Build history of the part. All positions in model axes, mm. A direction names the side the tool comes from. Round coordinates to 2 decimals unless told otherwise and drop trailing zeros. Order: outer loops, then holes, each group sorted by start corner. A loop starts at its lowest first (then second) coordinate and runs counter-clockwise, first axis right, second up. Notation, with made-up numbers: (71.25, -30.75) - (93.25, -30.75) arc R25 cw to (93.25, 7.25) - close; hole circle Ø1 at (41.25, 63). An arc over 180 degrees is marked (long way). One line per question, with ' | ' between items. Start each with the question number.
from build123d import *

# Parameters (mm, degrees)
SKETCH_1_R          = 11
SKETCH_1_R_2        = 5
EXTRUDE_1_DEPTH     = 6
SKETCH_2_R          = 9.499624375
SKETCH_2_R_2        = 7
CUT_EXTRUDE_1_DEPTH = 0.6
SKETCH_3_R          = 9.950876812
SKETCH_3_R_2        = 7
CUT_EXTRUDE_2_DEPTH = 0.6
CHAMFER_1_SIZE      = 0.2


with BuildPart() as part:
    # 草图1 → 凸台-拉伸1 (new body)
    with BuildSketch(Plane(origin=(0, 0, 0), x_dir=(0, 0, -1), z_dir=(1, 0, 0))):
        Circle(SKETCH_1_R)
        Circle(SKETCH_1_R_2, mode=Mode.SUBTRACT)
    extrude(amount=EXTRUDE_1_DEPTH)

    # 草图2 → 切除-拉伸1 (cut)
    with BuildSketch(Plane(origin=(6, 0, 0), x_dir=(0, 0, -1), z_dir=(1, 0, 0))):
        with Locations((-0.000375625, 0)):
            Circle(SKETCH_2_R)
        with Locations((-0.000375625, 0)):
            Circle(SKETCH_2_R_2, mode=Mode.SUBTRACT)
    extrude(amount=-CUT_EXTRUDE_1_DEPTH, mode=Mode.SUBTRACT)

    # 草图3 → 切除-拉伸2 (cut)
    with BuildSketch(Plane.ZY):
        with Locations((0.450876812, 0)):
            Circle(SKETCH_3_R)
        with Locations((0.450876812, 0)):
            Circle(SKETCH_3_R_2, mode=Mode.SUBTRACT)
    extrude(amount=-CUT_EXTRUDE_2_DEPTH, mode=Mode.SUBTRACT)

    # 倒角1
    chamfer_1_edges = [part.edges().sort_by_distance(p)[0] for p in [
        (0, 0, 11),
        (6, 0, 11),
        (0, 0, 5),
        (6, 0, 5),
    ]]
    chamfer(chamfer_1_edges, length=CHAMFER_1_SIZE)


solid = part.part
Item 1: Pull direction Z, two halves, no side cores. Call faces 1 (the face through (2.96, -10.74, 2.38)), 2 (the face through (6, -10, 0)), 3 (the face through (0.296, 9.866, -0.845)): released by +Z, released by -Z, zero draft, split by the parting line, or undercut.
Item 2: Wall check: line 1 along X through (y, z) = (-9, 2.5); line 2 along X through (y, z) = (4.25, -5.5); line 3 along Y through (x, z) = (0.5, -1). Give the ranges that are in metal, low to high. Write a range as [from, to].
Item 3: Slice it at C-C (x = 4.5). Write the cut outline in (y, z).
Item 4: 3-axis set-ups, long thin cutter, end or side, ignore diameter. For faces 4 (the face through (0, -1.5, 5.2)), 5 (the face through (0.3, 4.73, -4.71)), 6 (the face through (5.704, -3.638, -8.775)): which of +Z, -Z, +X, -X, +Y, -Y reach the whole face in a straight line?
Item 5: Pin check, flat tip, straight feed: pin 1 (8 mm diameter, centred on y = 0, z = 0, fed in from +X). Stop position of the tip, or through.
A:
1) face 1: split by the parting line | face 2: zero draft | face 3: undercut
2) line 1: [0.6, 5.4] | line 2: [0.6, 6] | line 3: [-10.95, -9.84], [-6.85, -4.9], [4.9, 6.85], [9.84, 10.95]
3) outline: circle Ø22 at (0, 0); hole circle Ø10 at (0, 0)
4) face 4: +Z, -Z, -X, +Y, -Y | face 5: -X | face 6: +X
5) pin 1: through
